Part print with two shaded views. Sizes in mm from the minimum x, y, z corner. A direction names the side the tool comes from. Coordinates: 2 decimals unless noted, no trailing zeros. Loops run counter-clockwise (first coordinate to the right, second up) from the corner with the lowest first, then second, coordinate; pieces in that order, holes last. Notation, with made-up numbers: (83, -28.5) -> (123, -28.5) arc R17 ccw to (123, -7.5) -> close; hole circle Ø1 at (77, -30). An arc over 180 degrees is marked (long way). Use one line per item in the form item = value.
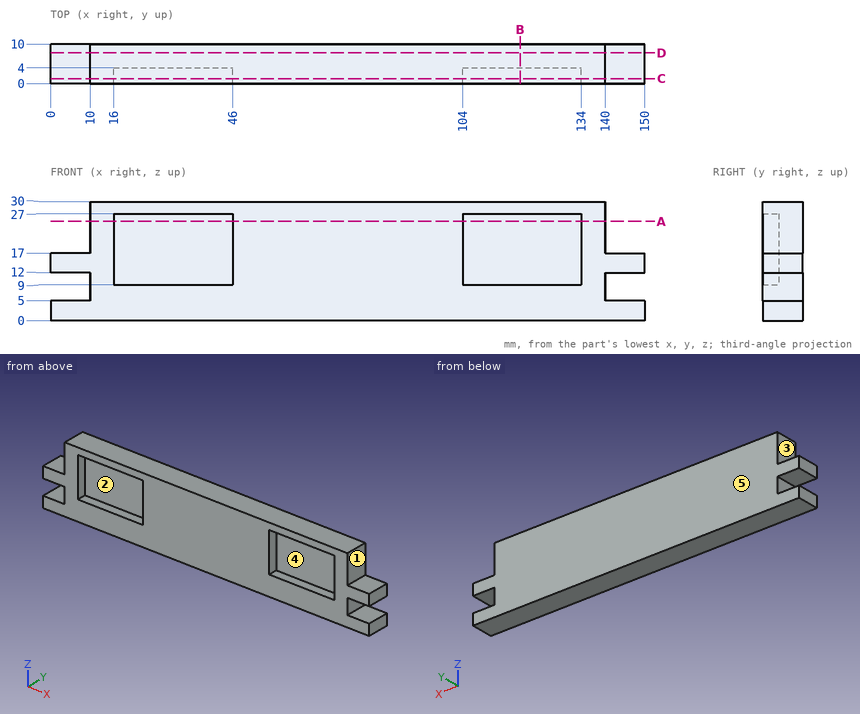
Q1. Band-saw the part on B-B, the plane x = 118.5. Write the cut outline in (y, z).
Result:
outline = (0, 0) -> (10, 0) -> (10, 30) -> (0, 30) -> (0, 27) -> (4, 27) -> (4, 9) -> (0, 9) -> close
Q2. Band-saw the part on A-A, the plane z = 25. Write the cut outline in (x, y).
Result:
outline = (10, 0) -> (16, 0) -> (16, 4) -> (46, 4) -> (46, 0) -> (104, 0) -> (104, 4) -> (134, 4) -> (134, 0) -> (140, 0) -> (140, 10) -> (10, 10) -> close
Q3. Mould opens along Z. For the marked faces 4 and 5 say: released by +Z, released by -Z, zero draft, split by the parting line, or undercut.
Result:
face_4 = undercut
face_5 = zero draft
Q4. Pin check, flat tips, straight feed: pin 1 Ø3 at (x, y) = (143.5, 4.5) entering from +Z; pin 2 Ø5.5 at (x, z) = (113, 19.5) entering from -Y; pin 3 Ø3.5 at (y, z) = (7, 8.5) entering from +X. Stop position of each tip, or through.
Result:
pin_1 = 17
pin_2 = 4
pin_3 = 140
Q5. Wall check: line 1 along X through (y, z) = (1, 14.5); line 2 along X through (y, z) = (3.75, 10); line 3 along Z through (x, y) = (125, 2.25). Give the ranges that are in metal, low to high.
Result:
line_1 = 0 to 16, 46 to 104, 134 to 150
line_2 = 10 to 16, 46 to 104, 134 to 140
line_3 = 0 to 9, 27 to 30
Q6. Band-saw the part on D-D, the plane y = 7.75. Write the cut outline in (x, z), and give its area (3 significant figures).
Result:
outline = (0, 0) -> (150, 0) -> (150, 5) -> (140, 5) -> (140, 12) -> (150, 12) -> (150, 17) -> (140, 17) -> (140, 30) -> (10, 30) -> (10, 17) -> (0, 17) -> (0, 12) -> (10, 12) -> (10, 5) -> (0, 5) -> close
area = 4,100 mm2
Q7. Band-saw the part on C-C, the plane y = 1.25. Write the cut outline in (x, z), and give its area (3 significant figures).
Result:
outline = (0, 0) -> (150, 0) -> (150, 5) -> (140, 5) -> (140, 12) -> (150, 12) -> (150, 17) -> (140, 17) -> (140, 30) -> (10, 30) -> (10, 17) -> (0, 17) -> (0, 12) -> (10, 12) -> (10, 5) -> (0, 5) -> close; hole (16, 9) -> (46, 9) -> (46, 27) -> (16, 27) -> close; hole (104, 9) -> (134, 9) -> (134, 27) -> (104, 27) -> close
area = 3,020 mm2
Q8. Which spindle directions (+Z, -Z, +X, -X, +Y, -Y) get a long thin tool onto all of the face, cutting with end or side? Do the marked faces 1, 2 and 3. Say none if no direction does.
Result:
face_1 = +Z, +X, +Y, -Y
face_2 = -Y
face_3 = +Z, -X, +Y, -Y
